Autodesk Inventor part; units mm, degrees
ref_plane "YZ Plane" through (0, 0, 0) normal (1, 0, 0) x (0, 1, 0)
ref_plane "XZ Plane" through (0, 0, 0) normal (0, 1, 0) x (-1, 0, 0)
ref_plane "XY Plane" through (0, 0, 0) normal (0, 0, 1) x (1, 0, 0)
sketch "스케치1" plane through (0, 0, 0) normal (0, 0, 1) x (1, 0, 0)
  line L0 (-4, -6) -> (4, -6)
  line L1 (4, -6) -> (4, 6)
  line L2 (4, 6) -> (-4, 6)
  line L3 (-4, 6) -> (-4, -6)
  line L4 (-4, -6) -> (4, 6) construction
  line L5 (4, -6) -> (-4, 6) construction
  line L6 (-6, 8) -> (-6, -8)
  line L7 (-6, -8) -> (6, -8)
  line L8 (6, -8) -> (6, 8)
  line L9 (6, 8) -> (4, 8)
  line L10 (4, 8) -> (4, 6)
  line L11 (-6, 8) -> (-4, 8)
  line L12 (-4, 8) -> (-4, 6)
  point P0 (0, 0)
  dimension "d0" = 8
  dimension "d1" = 12
  dimension "d2" = 2
  dimension "t" = 2
  dimension "d4" = 2
  dimension "d5" = 2
extrude "돌출1" add sketch "스케치1" along normal blind 7 contours L0 L1 L10 L9 L8 L7 L6 L11 L12 L3
sketch "스케치2" plane through (0, 0, 7) normal (0, 0, 1) x (1, 0, 0)
  line L0 (4, 8) -> (4, -6)
  line L1 (4, -6) -> (-4, -6)
  line L2 (-4, -6) -> (-4, 8)
  line L3 (-4, 8) -> (-6, 8)
  line L4 (-6, 8) -> (-6, -8)
  line L5 (-6, -8) -> (6, -8)
  line L6 (6, 8) -> (4, 8)
  line L7 (6, 8) -> (9, 8)
  line L8 (9, 8) -> (9, -8)
  line L9 (9, -8) -> (6, -8)
  point P0 (0, 0)
  dimension "d8" = 3
extrude "돌출2" add sketch "스케치2" along normal blind 1
sketch "스케치3" plane through (0, 0, 8) normal (0, 0, 1) x (1, 0, 0)
  line L0 (-6, 8) -> (-6, -8)
  line L1 (-6, -8) -> (9, -8)
  line L2 (9, -8) -> (9, 8)
  line L3 (9, 8) -> (4, 8)
  line L4 (4, 8) -> (4, -6)
  line L5 (4, -6) -> (-4, -6)
  line L6 (-4, -6) -> (-4, 8)
  line L7 (-4, 8) -> (-6, 8)
  line L8 (4, -6) -> (-4, -6)
  line L9 (4, -6) -> (7, -6)
  line L10 (7, -6) -> (7, 6)
  line L11 (7, 6) -> (4, 6)
  line L12 (4, 8) -> (4, -6)
  point P0 (0, 0)
  point P1 (4, 6)
  dimension "d11" = 2
  dimension "d12" = 2
extrude "돌출3" add sketch "스케치3" along normal blind 11 contours L7 L6 L5 L9 L10 L11 L4 L3 L2 L1 L0
sketch "스케치4" plane through (-4, -6, 0) normal (1, 0, 0) x (0, 0, -1)
  line L0 (-19, 0) -> (-19, 14)
  line L1 (0, 0) -> (-19, 0)
  line L2 (-19, 0) -> (-18, 0)
  line L3 (-18, 0) -> (-18, 5)
  line L4 (-18, 5) -> (-19, 5)
  line L5 (-19, 5) -> (-19, 0)
  point P0 (0, 6)
  dimension "d15" = 1
  dimension "d16" = 5
extrude "돌출4" add sketch "스케치4" along normal blind 2
ref_plane "작업 평면1" through (-6, 0, 0) normal (0, 1, 0) x (1, 0, 0)
sketch "스케치5" plane through (-6, 0, 0) normal (0, 1, 0) x (1, 0, 0)
  line L0 (0, 0) -> (12, 0)
  line L1 (12, 0) -> (12, -7)
  line L2 (12, -7) -> (15, -7)
  line L3 (15, -7) -> (15, -19)
  line L4 (0, -19) -> (15, -19)
  line L5 (0, 0) -> (0, -19)
  line L6 (0, 0) -> (0, -19)
  circle A0 centre (0, -13) radius 0.9
  line L7 (-0.6708, -12.4) -> (0, -12.4)
  point P0 (6, 0)
  point P1 (0, -13.9)
  dimension "k" = 1.8
  dimension "d20" = 0.6
  dimension "d21" = 6
extrude "돌출5" add sketch "스케치5" along normal mid plane 6 contours L5 A0 L7 picked at (-0.0684, -13.3921)
ref_plane "작업 평면2" through (1.5, -8, 0) normal (-1, 0, 0) x (0, 0, 1)
mirror "미러1" about plane through (1.5, -8, 0) normal (-1, 0, 0) of "돌출5"
fillet "모깎기1" radius 2 3 edges at (9, 8, 13) (-6, -8, 9.5) (9, -8, 13)
sketch "스케치6" plane through (4, 8, 0) normal (0, 1, 0) x (1, 0, 0)
  line L0 (0, 0) -> (0, -19)
  line L1 (0, -12) -> (1, -12)
  line L2 (1, -12) -> (1, -11.9)
  line L3 (1, -11.9) -> (0, -11.9)
  line L4 (0, -11.9) -> (0, -12)
  line L5 (3, -19) -> (0, -19)
  point P0 (-4, 0)
  point P1 (0, -11.9)
  dimension "d25" = 1
  dimension "d26" = 0.1
  dimension "d29" = 7
extrude "돌출6" cut sketch "스케치6" against normal up to surface (2 mm away)
chamfer "모따기1" distance 2 angle 45 1 edges at (4.5, 6, 12)
chamfer "모따기2" distance 1 angle 45 1 edges at (4.5, 8, 11.9)
equation "\"d2\" = t"
equation "\"d4\" = t"
properties part number "_3D 인쇄"
Geometry: final body of the model. Coordinates: model frame, mm. A direction names the side the tool comes from. Round coordinates to 2 decimals unless told otherwise and drop trailing zeros. Order: outer loops, then holes, each group sorted by start corner. A loop starts at its lowest first (then second) coordinate and runs counter-clockwise, first axis right, second up. Notation, with made-up numbers: M 85.5,-31.5 L 143.5,-31.5 A15 cw 143.5,-27.5 Z; hole C -8,-16 d2. An arc over 180 degrees is marked long. Use one line per item in the form item = value. Start each with the question number.
Q1. Pin query (flat end, axial travel): pin 1 Ø1 at (x, z) = (9, 13) entering from +Y; pin 2 Ø6 at (y, z) = (1.5, 17) entering from +X; pin 3 Ø3.5 at (y, z) = (3.5, 8) entering from -X; pin 4 Ø2 at (x, y) = (-0.5, -4.5) entering from -Z. Return the tip coordinate at first contact, or that it passes through.
Q2. Cut plane C-C (z = 4.75). Return loops of the section in (x, y), and give its area (3 significant figures).
Q3. Cut plane A-A (y = -4.75). Return loops of the section in (x, z), and give its area (3 significant figures).
Q4. Cut plane D-D (x = -3). Return loops of the section in (y, z).
Q5. Material intervals for line 1 (X direction, y = -3.75, z = 16.5); line 2 (X direction, y = -4.5, z = 2); line 3 (Y direction, x = 4.5, z = 9.75), sorted ascending. Write a range as [from, to].
Q6. Access query for faces 5 (the face through (-4, 1, 9)), 6 (the face through (0, -6, 9)), 7 (the face through (9.4, -3, 13.1)). Directions: +Z, -Z, +X, -X, +Y, -Y. A direction counts if a zero-diameter tool reaches every point of the face in a straight line with its end or side. Return the directions, or none.
Q7. Mould query, pull axis Z, two halves, no side actions, for faces 1 (the face through (4.5, 7, 13)), 2 (the face through (-2, -3.5, 18.5)), 3 (the face through (5, 0, 8)), 4 (the face through (-6.816, -0.042, 13.381)). Classes: +Z half, -Z half, draft (parallel to the pull), parting line (faces both ways), or undercut.
Geometry results:
q1.pin_1 = 7.32
q1.pin_2 = 9
q1.pin_3 = -6
q1.pin_4 = through
q2.outline = M -6,-6 A2 ccw -4,-8 L 6,-8 L 6,8 L 4,8 L 4,-6 L -4,-6 L -4,8 L -6,8 Z
q2.area = 79.1 mm^2
q3.outline = M -6,0 L -4,0 L -4,18 L -2,18 L -2,19 L -6,19 Z; M 4,0 L 6,0 L 6,7 L 9,7 L 9,19 L 7,19 L 7,8 L 4,8 Z
q3.area = 81.0 mm^2
q4.outline = M -8,0 L -6,0 L -6,18 L -1,18 L -1,19 L -8,19 Z
q5.line_1 = [-6, -4], [7, 9]
q5.line_2 = [-6, -4], [4, 6]
q5.line_3 = [-8, -6], [6, 8]
q6.face_5 = -Z, +Y
q6.face_6 = none
q6.face_7 = +Z, -Z, +X, -Y
q7.face_1 = undercut
q7.face_2 = draft
q7.face_3 = +Z half
q7.face_4 = parting line
